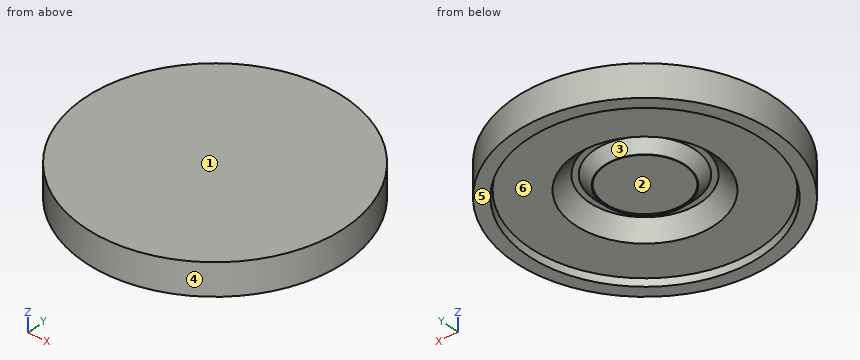
Autodesk Inventor part; units mm, degrees
ref_plane "YZ Plane" through (0, 0, 0) normal (1, 0, 0) x (0, 1, 0)
ref_plane "XZ Plane" through (0, 0, 0) normal (0, 1, 0) x (-1, 0, 0)
ref_plane "XY Plane" through (0, 0, 0) normal (0, 0, 1) x (1, 0, 0)
sketch "Skizze1" plane through (0, 0, 0) normal (1, 0, 0) x (0, 1, 0)
  line L0 (5, 0) -> (-30, 0)
  line L1 (5, -3) -> (5, 0)
  line L2 (-3.9492, 2.2) -> (-21.0508, 2.2)
  line L3 (-6.3, 0.7) -> (-18.7, 0.7)
  line L4 (-12.5, 0.7) -> (-12.5, 5.3428)
  line L5 (5, 0) -> (-2.1515, 0)
  line L6 (-18.5, 0.7) -> (-6.5, 0.7) construction
  line L7 (-6.5, 0.7) -> (-6.5, 0.9) construction
  line L8 (-6.5, 0.9) -> (-18.5, 0.9) construction
  line L9 (-18.5, 0.9) -> (-18.5, 0.7) construction
  line L10 (-18.5, 0.7) -> (-6.5, 0.9) construction
  line L11 (-6.5, 0.7) -> (-18.5, 0.9) construction
  line L12 (-6.3, 0.7) -> (-7.4658, 0.7) construction
  line L13 (-12.5, 0.9) -> (-6.4, 0.9)
  line L14 (-6.4, 0.9) -> (-6.4, 0.7)
  line L15 (-6.3, 0.7) -> (-6.4, 0.7)
  line L16 (-12.5, 0.9) -> (-12.5, 3.9)
  line L17 (-12.5, 3.9) -> (5, 3.9)
  line L18 (5, 3.9) -> (5, 0)
  line L19 (-4.8, 2.2) -> (-6.3, 0.7)
  line L20 (-3.9492, 2.2) -> (-21.0508, 2.2)
  line L21 (-1.7515, 0) -> (-3.9503, 2.1989)
  line L22 (-5.7431, 0.4) -> (-4.5431, 1.6) construction
  line L23 (-4.1977, 1.6) -> (-20.8023, 1.6) construction
  line L24 (-4.1977, 1.6) -> (-3.1977, 0.6) construction
  line L25 (-4.1977, 1.6) -> (-20.8023, 1.6) construction
  line L26 (5, 3.9) -> (7.4806, 3.9)
  line L27 (7.4806, 3.9) -> (7.4806, -1.0263)
  line L28 (7.4806, -1.0263) -> (5.458, -1.0263)
  line L29 (5, 0) -> (5.2, 0)
  line L30 (5.2, 0) -> (5.4633, -1.0263)
  point P0 (0, 0)
  point P1 (-5.8, 2.2)
  point P2 (-12.5, 0.8)
  point P3 (-12.5, 0.9)
  point P4 (-1.7515, 0)
  dimension "d0" = 12
  dimension "d1" = 0.2
  dimension "d2" = 6.1
  dimension "d3" = 3
  dimension "d5" = 0.2
revolve "Umdrehung1" add sketch "Skizze1" angle 360 about axis through (0, -12.5, 0.7) along (0, 0, 1) contours L0 L21 L2 L4 L17 L18 | L18 L26 L27 L28 L30 L29 | L19 L3 L14 L13 L4 L2
properties part number "50_ETL_Membrane_Mould_Upper_v0"
Work out the finished part from the listing and answer in its coordinate system (mm). Face numbers are marked on the shaded views. A direction names the side the tool comes from. Give positions to 0.01 mm unless a question says otherwise; leave off trailing zeros. Write each loop counter-clockwise with the first axis right and the second up, starting at its lowest first coordinate (ties: lowest second). Pieces come first, ordered by that corner, then holes. Notation, with made-up numbers: (-18, 38) -> (20, 38) arc R24 ccw to (20, 48) -> close; hole circle Ø9 at (-5, 34.5). An arc over 180 degrees is marked (long way). Write item = value, one per line.
Q1. Flat-ended cylindrical pins translate along their axes: pin 1 Ø2 at (x, z) = (-10.5, 0.5) entering from -Y; pin 2 Ø3.5 at (x, y) = (2.5, -14) entering from -Z; pin 3 Ø10 at (x, y) = (1.5, -10) entering from -Z. Find the tip coordinate at first contact, or state that the pin passes through.
Computed values:
pin_1 = -30.08
pin_2 = 0.9
pin_3 = 0.7
Q2. For a pull along X with two mould halves and no side action, classify the marked faces 1, 2, 3 and 4 as pulls with the +X half, pulls with the -X half, needs draft (parallel to the pull), parting line crosses it, or undercut.
Computed values:
face_1 = needs draft
face_2 = undercut
face_3 = undercut
face_4 = parting line crosses it
Q3. Section A-A on y = -12.5 is taken. Determine the outline of the cut face in (x, z).
Computed values:
outline = (-19.98, -1.03) -> (-17.96, -1.03) -> (-17.7, 0) -> (-10.75, 0) -> (-8.55, 2.2) -> (-7.7, 2.2) -> (-6.2, 0.7) -> (-6.1, 0.7) -> (-6.1, 0.9) -> (6.1, 0.9) -> (6.1, 0.7) -> (6.2, 0.7) -> (7.7, 2.2) -> (8.55, 2.2) -> (10.75, 0) -> (17.7, 0) -> (17.96, -1.03) -> (19.98, -1.03) -> (19.98, 3.9) -> (-19.98, 3.9) -> close
Q4. A tool of negligible diameter and unlimited length cuts with its end or side. For the marked faces 5 and 6, from which of +Z, -Z, +X, -X, +Y, -Y can it reach the whole face along a straight path? Write none if from no direction.
Computed values:
face_5 = -Z, +X, -X, +Y, -Y
face_6 = -Z
Q5. Consider line 1 along X through (y, z) = (-12.5, 0.8); line 2 along Y through (x, z) = (0, 0.8); line 3 along Y through (x, z) = (-6, 1.35). Determine where each line is inside the solid, lowest interval first.
Computed values:
line_1 = -19.98 to -9.95, -6.3 to -6.1, 6.1 to 6.3, 9.95 to 19.98
line_2 = -32.48 to -22.45, -18.8 to -18.6, -6.4 to -6.2, -2.55 to 7.48
line_3 = -31.56 to -19.74, -15.8 to -9.2, -5.26 to 6.56
Q6. Section C-C on z = 1.6 is taken. Determine the outline of the cut face in (x, y), and give its area (3 significant figures).
Computed values:
outline = circle Ø39.96 at (0, -12.5); circle Ø14.2 at (0, -12.5); hole circle Ø18.3 at (0, -12.5)
area = 1,150 mm^2
Q7. Section B-B on x = 0 is taken. Determine the outline of the cut face in (y, z).
Computed values:
outline = (-32.48, -1.03) -> (-30.46, -1.03) -> (-30.2, 0) -> (-23.25, 0) -> (-21.05, 2.2) -> (-20.2, 2.2) -> (-18.7, 0.7) -> (-18.6, 0.7) -> (-18.6, 0.9) -> (-6.4, 0.9) -> (-6.4, 0.7) -> (-6.3, 0.7) -> (-4.8, 2.2) -> (-3.95, 2.2) -> (-1.75, 0) -> (5.2, 0) -> (5.46, -1.03) -> (7.48, -1.03) -> (7.48, 3.9) -> (-32.48, 3.9) -> close
Q8. Section D-D on z = -0.55 is taken. Determine the outline of the cut face in (x, y).
Computed values:
outline = circle Ø39.96 at (0, -12.5); hole circle Ø35.68 at (0, -12.5)
